Build history of the part. All positions in model axes, mm. A direction names the side the tool comes from. Round coordinates to 2 decimals unless told otherwise and drop trailing zeros. Order: outer loops, then holes, each group sorted by start corner. A loop starts at its lowest first (then second) coordinate and runs counter-clockwise, first axis right, second up. Notation, with made-up numbers: (-5.75, 67.25) -> (14.25, 67.25) arc R20 ccw to (14.25, 101.25) -> close; hole circle Ø2 at (25.5, -26.5). An arc over 180 degrees is marked (long way). Answer as a JSON object with one key per item and string values.
from build123d import *

# Parameters (mm, degrees)
BOSS_EXTRUDE1_DEPTH = 10
CUT_EXTRUDE1_DEPTH  = 102.942524855
SKETCH15_R          = 2.2
CUT_EXTRUDE5_DEPTH  = 20.069609228
CUT_EXTRUDE6_DEPTH  = 15
CUT_EXTRUDE7_DEPTH  = 15
BOSS_EXTRUDE2_DEPTH = 9
SKETCH21_W          = 10
SKETCH21_H          = 7.31662479
BOSS_EXTRUDE3_DEPTH = 1
SKETCH17_R          = 2.2
CUT_EXTRUDE8_DEPTH  = 11
SKETCH22_R          = 3.5
CUT_EXTRUDE9_DEPTH  = 4
SKETCH23_R          = 2.2
BOSS_EXTRUDE4_DEPTH = 1


with BuildPart() as part:
    # Sketch1 → Boss-Extrude1 (new body)
    with BuildSketch(Plane(origin=(0, 0, 0), x_dir=(1, 0, 0), z_dir=(0, 1, 0))):
        Polygon((-5, 19.95), (7.9685, 33.8358924), (7.9685, 50.971262428), (18.4685, 50.971262428), (18.4685, 34.371262428), (5, 19.95), (5, -19.95), (18.4685, -34.371262428), (18.4685, -50.971262428), (7.9685, -50.971262428), (7.9685, -33.8358924), (-5, -19.95), align=None)
    extrude(amount=BOSS_EXTRUDE1_DEPTH)

    # Sketch2 → Cut-Extrude1 (cut, through all)
    with BuildSketch(Plane.XY.offset(50.971262428)):
        Polygon((11.9685, 10), (18.4685, 3.5), (18.4685, 10), align=None)
    extrude(amount=-CUT_EXTRUDE1_DEPTH, mode=Mode.SUBTRACT)

    # Sketch15 → Cut-Extrude5 (cut, through all)
    with BuildSketch(Plane(origin=(10.98425, 10.98425, 0), x_dir=(0, 0, -1), z_dir=(0.707106781, 0.707106781, 0))):
        with Locations(Location((44.471262428, -5.685327854, 0), (0, 0, 90))):  # turned: the seam where the file's is
            Circle(SKETCH15_R)
        with Locations(Location((-44.471262428, -5.685327854, 0), (0, 0, 178.678239242))):  # turned: the seam where the file's is
            Circle(SKETCH15_R)
    extrude(amount=-CUT_EXTRUDE5_DEPTH, mode=Mode.SUBTRACT)

    # Sketch4 → Cut-Extrude6 (cut)
    with BuildSketch(Plane.XY.offset(50.971262428)):
        Polygon((7.9685, 4.949747468), (7.9685, 0), (12.918247468, 0), align=None)
    extrude(amount=-CUT_EXTRUDE6_DEPTH, mode=Mode.SUBTRACT)

    # Sketch18 → Cut-Extrude7 (cut)
    with BuildSketch(Plane(origin=(0, 0, -50.971262428), x_dir=(-1, 0, 0), z_dir=(0, 0, -1))):
        Polygon((-7.9685, 5), (-7.9685, 0), (-12.918247468, 0), align=None)
    extrude(amount=-CUT_EXTRUDE7_DEPTH, mode=Mode.SUBTRACT)

    # Sketch13 → Boss-Extrude2 (add)
    with BuildSketch(Plane(origin=(5, 0, 0), x_dir=(0, 0, -1), z_dir=(1, 0, 0))):
        Polygon((0, 7.31662479), (-5, 4), (-5, 0), (5, 0), (5, 4), align=None)
    extrude(amount=BOSS_EXTRUDE2_DEPTH)

    # Sketch21 → Boss-Extrude3 (add)
    with BuildSketch(Plane(origin=(14, 0, 0), x_dir=(0, 0, -1), z_dir=(1, 0, 0))):
        with Locations((0, 3.658312395)):
            Rectangle(SKETCH21_W, SKETCH21_H)
    extrude(amount=BOSS_EXTRUDE3_DEPTH)

    # Sketch17 → Cut-Extrude8 (cut, through all)
    with BuildSketch(Plane(origin=(0, 10, 0), x_dir=(1, 0, 0), z_dir=(0, 1, 0))):
        with Locations(Location((0, 12, 0), (0, 0, 270))):  # turned: the seam where the file's is
            Circle(SKETCH17_R)
        with Locations(Location((0, -12, 0), (0, 0, 270))):  # turned: the seam where the file's is
            Circle(SKETCH17_R)
    extrude(amount=-CUT_EXTRUDE8_DEPTH, mode=Mode.SUBTRACT)

    # Sketch22 → Cut-Extrude9 (cut)
    with BuildSketch(Plane.XZ):
        with Locations(Location((0, 12, 0), (0, 0, 270))):  # turned: the seam where the file's is
            Circle(SKETCH22_R)
        with Locations(Location((0, -12, 0), (0, 0, 270))):  # turned: the seam where the file's is
            Circle(SKETCH22_R)
    extrude(amount=-CUT_EXTRUDE9_DEPTH, mode=Mode.SUBTRACT)

    # Sketch23 → Boss-Extrude4 (add)
    with BuildSketch(Plane(origin=(0, 10, 0), x_dir=(1, 0, 0), z_dir=(0, 1, 0))):
        Polygon((5, -30.657400548), (5, 30.657400548), (-5, 19.95), (-5, -19.95), align=None)
        with Locations(Location((0, -12, 0), (0, 0, 270))):  # turned: the seam where the file's is
            Circle(SKETCH23_R, mode=Mode.SUBTRACT)
        with Locations(Location((0, 12, 0), (0, 0, 270))):  # turned: the seam where the file's is
            Circle(SKETCH23_R, mode=Mode.SUBTRACT)
    extrude(amount=BOSS_EXTRUDE4_DEPTH)


solid = part.part
1) Pull direction Y, two halves, no side cores. Call faces 1 (the face through (13.11, 4.4, -46.62)), 2 (the face through (2, 4, 10)), 3 (the face through (18.468, 2, 43)): pulls with the +Y half, pulls with the -Y half, needs draft (parallel to the pull), parting line crosses it, or undercut.
Checked values:
{"face 1": "undercut", "face 2": "pulls with the -Y half", "face 3": "needs draft"}
2) Cut at C-C, the plane z = -19. Give the cut face in (x, y).
Checked values:
{"outline": "(-5, 0) -> (5, 0) -> (5, 11) -> (-5, 11) -> close"}
3) Flat gauge pins, fed straight in: pin 1 Ø2.5 at (x, z) = (0, -12) entering from +Y; pin 2 Ø2 at (y, z) = (5, -1.5) entering from +X; pin 3 Ø5.5 at (x, z) = (7.5, 40.5) entering from +Y; pin 4 Ø2 at (x, z) = (1, -11) entering from -Y. Where does each tip first touch, or does it go through?
Checked values:
{"pin 1": "passes through", "pin 2": "stops at x = 15", "pin 3": "stops at y = 10", "pin 4": "stops at y = 4"}
4) Which spindle directions (+Z, -Z, +X, -X, +Y, -Y) get a long thin tool onto all of the face, cutting with end or side? Do faces 4 (the face through (0.154, 1.972, -8.503)), 5 (the face through (10.332, 4.93, -25.659)), 6 (the face through (7.968, 7, 43)), 7 (the face through (9, 1, 35.971)). Say none if no direction does.
Checked values:
{"face 4": "-Y", "face 5": "+X, +Y, -Y", "face 6": "+Z, -X, +Y, -Y", "face 7": "+Z, -X, -Y"}
5) Probe L1, parallel to X at y = 10.3, z = -12; L2, parallel to Z at x = 0.25, y = 6.25; L3, parallel to X at y = 5.5, z = -4.5. List the from-to ranges inside material, lowest first. Write a range as from..to.
Checked values:
{"L1": "x = -5..-2.2, 2.2..5", "L2": "z = -25.57..-14.19, -9.81..9.81, 14.19..25.57", "L3": "x = -5..5, 14..15"}
6) Cut at A-A, the plane z = 12. Give the cut face in (x, y).
Checked values:
{"outline": "(-5, 0) -> (-3.5, 0) -> (-3.5, 4) -> (-2.2, 4) -> (-2.2, 11) -> (-5, 11) -> close; (2.2, 4) -> (3.5, 4) -> (3.5, 0) -> (5, 0) -> (5, 11) -> (2.2, 11) -> close"}
7) Cut at B-B, the plane z = 40. Give the cut face in (x, y), plus the area to 3 significant figures.
Checked values:
{"outline": "(7.97, 4.95) -> (12.92, 0) -> (18.47, 0) -> (18.47, 3.5) -> (11.97, 10) -> (7.97, 10) -> close", "area": "71.6 mm²"}
